from build123d import *

# Parameters (mm, degrees)
SKETCH1_W           = 300
SKETCH1_H           = 40
BOSS_EXTRUDE1_DEPTH = 10
SKETCH2_R           = 7.5
BOSS_EXTRUDE2_DEPTH = 30
SKETCH3_W           = 40
SKETCH3_H           = 40
BOSS_EXTRUDE3_DEPTH = 40
SKETCH4_W           = 60
SKETCH4_H           = 20
CUT_EXTRUDE1_DEPTH  = 58


with BuildPart() as part:
    # Sketch1 → Boss-Extrude1 (new, symmetric)
    with BuildSketch(Plane.XY):
        Rectangle(SKETCH1_W, SKETCH1_H)
    extrude(amount=BOSS_EXTRUDE1_DEPTH, both=True)

    # Sketch2 → Boss-Extrude2 (add, symmetric)
    with BuildSketch(Plane.XY):
        with Locations((-135, 0)):
            Circle(SKETCH2_R)
    extrude(amount=BOSS_EXTRUDE2_DEPTH, both=True)

    # Sketch3 → Boss-Extrude3 (add)
    with BuildSketch(Plane(origin=(150, 0, 0), x_dir=(0, 0, -1), z_dir=(1, 0, 0))):
        Rectangle(SKETCH3_W, SKETCH3_H)
    extrude(amount=BOSS_EXTRUDE3_DEPTH)

    # Sketch4 → Cut-Extrude1 (cut)
    with BuildSketch(Plane.XY.offset(20)):
        with Locations((190, 0)):
            Rectangle(SKETCH4_W, SKETCH4_H)
    extrude(amount=-CUT_EXTRUDE1_DEPTH, mode=Mode.SUBTRACT)


solid = part.part
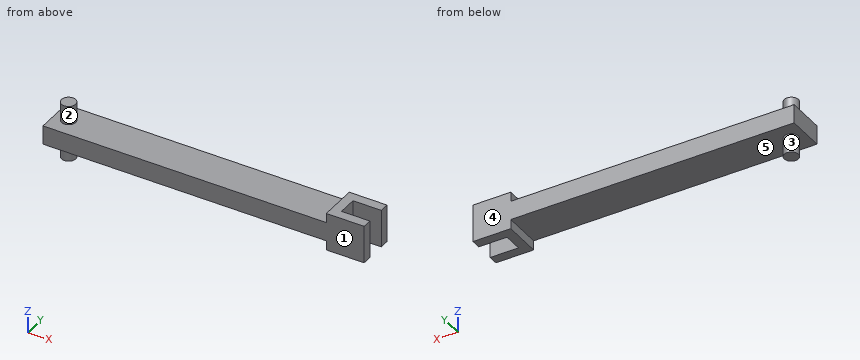
Geometry check sheet. Reference: the model listing, model coordinates, mm. Face numbers are marked on the shaded views. A direction names the side the tool comes from. Give positions to 0.01 mm unless a question says otherwise; leave off trailing zeros. Write each loop counter-clockwise with the first axis right and the second up, starting at its lowest first coordinate (ties: lowest second). Pieces come first, ordered by that corner, then holes. Notation, with made-up numbers: M 32,23.5 L 71,23.5 A23 cw 71,37.5 Z; hole C -28.5,16.25 d3. An arc over 180 degrees is marked long. One line per question, with ' | ' between items.
1. Gauge pin test, flat ends, axial feed: pin 1 (12 mm diameter, centred on x = 59, y = -7, fed in from -Z); pin 2 (4 mm diameter, centred on y = 4.5, z = -13.5, fed in from +X); pin 3 (20 mm diameter, centred on x = -17.5, y = -3.5, fed in from +Z). Record the tip position at first contact, or that the pin passes through.
Ans:
pin 1: z = -10 | pin 2: x = 160 | pin 3: z = 10
2. Mould release check, pull along X, two halves, no side actions. Record for the marked faces 4 and 5: released by +X, released by -X, zero draft, split by the parting line, or undercut.
Ans:
face 4: zero draft | face 5: undercut
3. Cross-section at D-D (y = 0). Enter the section's corners in (x, z), plus the area to 3 significant figures.
Ans:
outline: M -150,-10 L -142.5,-10 L -142.5,-30 L -127.5,-30 L -127.5,-10 L 150,-10 L 150,-20 L 160,-20 L 160,20 L 150,20 L 150,10 L -127.5,10 L -127.5,30 L -142.5,30 L -142.5,10 L -150,10 Z | area: 7,000 mm2
4. Scan lines: line 1 along Z through (x, y) = (162.5, -17); line 2 along Y through (x, z) = (174.5, -4); line 3 along X through (y, z) = (-9, -15). Record each from-to range of solid material in increasing order. Write a range as from..to.
Ans:
line 1: -20..20 | line 2: -20..-10, 10..20 | line 3: 150..160
5. Cross-section at C-C (y = 15). Enter the section's corners in (x, z), plus the area to 3 significant figures.
Ans:
outline: M -150,-10 L 150,-10 L 150,-20 L 190,-20 L 190,20 L 150,20 L 150,10 L -150,10 Z | area: 7,600 mm2
6. Cross-section at A-A (z = -6). Enter the section's corners in (x, y).
Ans:
outline: M -150,-20 L 190,-20 L 190,-10 L 160,-10 L 160,10 L 190,10 L 190,20 L -150,20 Z
7. Set-up check for the marked faces 1, 2 and 3: record each of +Z, -Z, +X, -X, +Y, -Y from which the full face is reachable in a straight line by a thin tool's end or side.
Ans:
face 1: +Z, -Z, +X, -X, -Y | face 2: +Z | face 3: -Z
8. Cross-section at B-B (x = -135). Enter the section's corners in (y, z), plus the area to 3 significant figures.
Ans:
outline: M -20,-10 L -7.5,-10 L -7.5,-30 L 7.5,-30 L 7.5,-10 L 20,-10 L 20,10 L 7.5,10 L 7.5,30 L -7.5,30 L -7.5,10 L -20,10 Z | area: 1,400 mm2
